Here's the drawing with two shaded views (mm, measured from the low corner). I have some questions. A direction names the side the tool comes from. Round coordinates to 2 decimals unless told otherwise and drop trailing zeros. Order: outer loops, then holes, each group sorted by start corner. A loop starts at its lowest first (then second) coordinate and runs counter-clockwise, first axis right, second up.
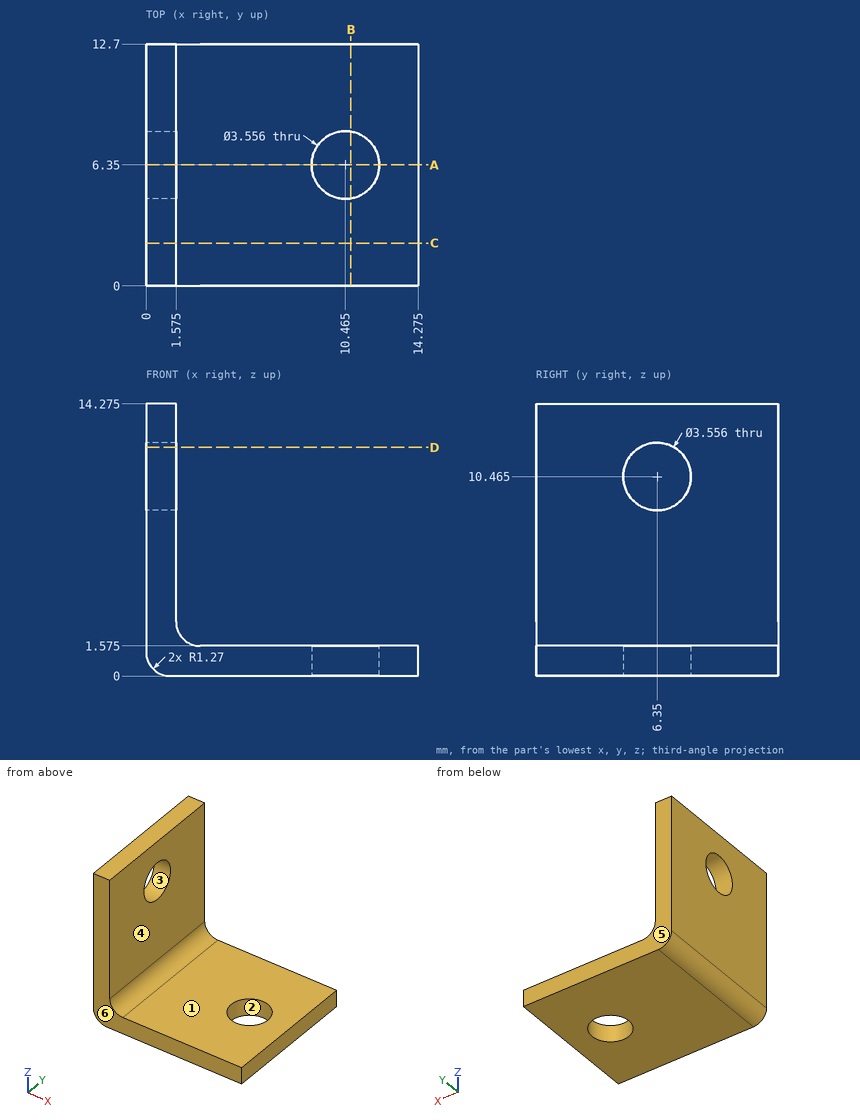
Q1. For P1, Ø3.5, axis at y = 5, z = 6.5, coming from the +X side (3 decimals); P2, Ø3.5, axis at x = 6, y = 7, coming from the +Z side (3 decimals), each with a flat end and sliding along its axis, tell me the tip position at first contact or that it passes through.
Q2. Imagine slicing it at A-A, the plane y = 6.35. Please give me the cut outline in (x, z) (1 decimal), then the cut area to 3 significant figures.
Q3. Imagine slicing it at C-C, the plane y = 2.25. Please give me the cut outline in (x, z) (1 decimal), then the cut area to 3 significant figures.
Q4. Imagine slicing it at B-B, the plane x = 10.75. Please give me the cut outline in (y, z) (1 decimal).
Q5. For the marked faces 1 and 2, which set-ups out of +Z, -Z, +X, -X, +Y, -Y let a thin tool reach every point of the face, with its end or its side?
Q6. I need wall thicknesses on L1, parallel to Z at x = 12.75, y = 8.5 (1 decimal); L2, parallel to Y at x = 1.25, z = 10.25 (1 decimal). Which ranges of each line are inside material? Lowest first, please.
Q7. Imagine slicing it at D-D, the plane z = 12. Please give me the cut outline in (x, y) (1 decimal).
Q8. We'd pull the mould along Y, two halves only. Please class the marked faces 3, 4, 5 and 6: released by +Y, released by -Y, zero draft, split by the parting line, or undercut.
Filled in:
1. P1: stops at x = 1.575
1. P2: stops at z = 1.575
2. outline: (0, 1.3) arc R1.3 ccw to (1.3, 0) - (8.7, 0) - (8.7, 1.6) - (2.8, 1.6) arc R1.3 cw to (1.6, 2.8) - (1.6, 8.7) - (0, 8.7) - close; (0, 12.2) - (1.6, 12.2) - (1.6, 14.3) - (0, 14.3) - close; (12.2, 0) - (14.3, 0) - (14.3, 1.6) - (12.2, 1.6) - close
2. area: 31.3 mm2
3. outline: (0, 1.3) arc R1.3 ccw to (1.3, 0) - (14.3, 0) - (14.3, 1.6) - (2.8, 1.6) arc R1.3 cw to (1.6, 2.8) - (1.6, 14.3) - (0, 14.3) - close
3. area: 42.5 mm2
4. outline: (0, 0) - (4.6, 0) - (4.6, 1.6) - (0, 1.6) - close; (8.1, 0) - (12.7, 0) - (12.7, 1.6) - (8.1, 1.6) - close
5. face 1: +Z, +X, +Y, -Y
5. face 2: +Z, -Z
6. L1: z = 0 to 1.6
6. L2: y = 0 to 4.6, 8.1 to 12.7
7. outline: (0, 0) - (1.6, 0) - (1.6, 5.5) - (0, 5.5) - close; (0, 7.2) - (1.6, 7.2) - (1.6, 12.7) - (0, 12.7) - close
8. face 3: undercut
8. face 4: zero draft
8. face 5: released by +Y
8. face 6: released by -Y
